Part model, mm, in its own coordinate system. Face numbers are marked on the shaded views. A direction names the side the tool comes from. Round coordinates to 2 decimals unless told otherwise and drop trailing zeros. Order: outer loops, then holes, each group sorted by start corner. A loop starts at its lowest first (then second) coordinate and runs counter-clockwise, first axis right, second up. Notation, with made-up numbers: (-33, 23) - (12, 23) arc R11 ccw to (12, 36) - close; hole circle Ø9 at (-14, -7). An arc over 180 degrees is marked (long way). Answer as a JSON object with one key per item and string values.
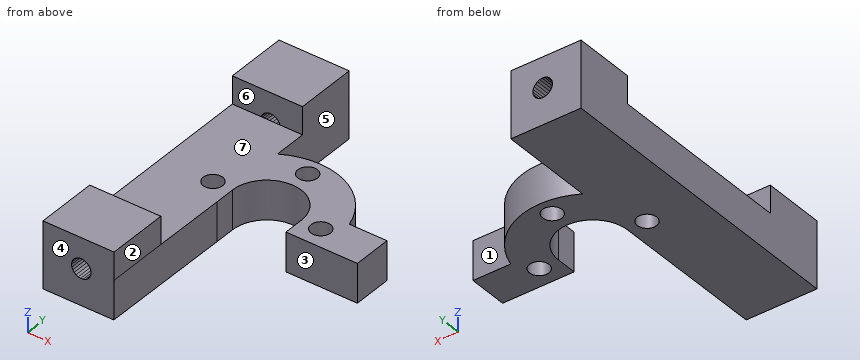
```python
from build123d import *

# Parameters (mm, degrees)
SKETCH1_R           = 1.5
BOSS_EXTRUDE1_DEPTH = 6
SKETCH2_W           = 10.807687298
SKETCH2_H           = 9.5
SKETCH2_W_2         = 10.943994224
BOSS_EXTRUDE2_DEPTH = 4.25
CUT_EXTRUDE1_DEPTH  = 9.5
CUT_EXTRUDE2_DEPTH  = 9.5


with BuildPart() as part:
    # Sketch1 → Boss-Extrude1 (new body)
    with BuildSketch(Plane.XY.offset(84.451608182)):
        with BuildLine():
            Line((40.02344809, 11.701998712), (40.02344809, 8.566491131))
            Line((40.02344809, 8.566491131), (47.02344809, 8.566491131))
            Line((47.02344809, 8.566491131), (51.02344809, 8.566491131))
            Line((51.02344809, 8.566491131), (51.02344809, 14.59568261))
            Line((51.02344809, 14.59568261), (45.222644144, 14.59568261))
            ThreePointArc((45.222644144, 14.59568261), (38.830062222, 21.788734788), (29.231135388, 21.10630759))
            Line((29.231135388, 21.10630759), (29.231135388, 35.703275576))
            Line((29.231135388, 35.703275576), (18.42344809, 35.703275576))
            Line((18.42344809, 35.703275576), (18.42344809, 14.59568261))
            Line((18.42344809, 14.59568261), (18.42344809, 8.566491131))
            Line((18.42344809, 8.566491131), (18.42344809, -12.296724841))
            Line((18.42344809, -12.296724841), (29.320619754, -12.296724841))
            Line((29.320619754, -12.296724841), (29.42344809, 8.566491131))
            Line((29.42344809, 8.566491131), (29.42344809, 11.701998712))
            ThreePointArc((29.42344809, 11.701998712), (34.72344809, 17.001998712), (40.02344809, 11.701998712))
        make_face()
        with Locations((43.02344809, 11.701998712)):
            Circle(SKETCH1_R, mode=Mode.SUBTRACT)
        with Locations((26.42344809, 11.701998712)):
            Circle(SKETCH1_R, mode=Mode.SUBTRACT)
        with Locations((34.72344809, 20.001998712)):
            Circle(SKETCH1_R, mode=Mode.SUBTRACT)
    extrude(amount=BOSS_EXTRUDE1_DEPTH)

    # Sketch2 → Boss-Extrude2 (add)
    with BuildSketch(Plane.XY.offset(90.451608182)):
        with Locations((23.827291739, 30.953275576)):
            Rectangle(SKETCH2_W, SKETCH2_H)
        with Locations((23.895445202, -7.546724841)):
            Rectangle(SKETCH2_W_2, SKETCH2_H)
    extrude(amount=BOSS_EXTRUDE2_DEPTH)

    # Sketch3 → Cut-Extrude1 (cut)
    with BuildSketch(Plane(origin=(0, 35.703275576, 0), x_dir=(1, 0, 0), z_dir=(0, 1, 0))):
        Polygon((24.039543919, -91.507423883), (24.414807311, -91.53103291), (24.784140042, -91.460577426), (25.124363355, -91.300484473), (25.414071731, -91.060813265), (25.635078303, -90.756623289), (25.773495189, -90.407027611), (25.820620111, -90.033992408), (25.773495189, -89.660958601), (25.635078303, -89.311362458), (25.414071731, -89.007172948), (25.124363355, -88.767500808), (24.784140042, -88.607407389), (24.414807311, -88.536952836), (24.039543919, -88.560561864), (23.681945852, -88.676751805), (23.364484064, -88.878222024), (23.107096306, -89.152314914), (22.925957791, -89.481805665), (22.832445554, -89.845992839), (22.832445554, -90.221992442), (22.925957791, -90.586179616), (23.107096306, -90.915670833), (23.364484064, -91.189762792), (23.681945852, -91.391233476), align=None)
    extrude(amount=-CUT_EXTRUDE1_DEPTH, mode=Mode.SUBTRACT)

    # Sketch4 → Cut-Extrude2 (cut)
    with BuildSketch(Plane.XZ.offset(12.296724841)):
        Polygon((25.27675753, 88.878222024), (24.959288291, 88.676751805), (24.601690225, 88.560561864), (24.226434282, 88.536952836), (23.857094101, 88.607407389), (23.516878239, 88.767500808), (23.227169863, 89.007172948), (23.00615584, 89.311362458), (22.867746405, 89.660958601), (22.820621482, 90.033992408), (22.867746405, 90.407027611), (23.00615584, 90.756623289), (23.227169863, 91.060813265), (23.516878239, 91.300484473), (23.857094101, 91.460577426), (24.226434282, 91.53103291), (24.601690225, 91.507423883), (24.959288291, 91.391233476), (25.27675753, 91.189762792), (25.534145287, 90.915670833), (25.715283803, 90.586179616), (25.80879604, 90.221992442), (25.80879604, 89.845992839), (25.715283803, 89.481805665), (25.534145287, 89.152314914), align=None)
    extrude(amount=-CUT_EXTRUDE2_DEPTH, mode=Mode.SUBTRACT)


solid = part.part
```
Item 1: Tool access for the marked faces 1, 2 and 3: list every direction of +Z, -Z, +X, -X, +Y, -Y with a clear straight run to the whole face (end or side of a thin tool).
Taken from the geometry:
{"face 1": "+Z, -Z, +X, +Y", "face 2": "+Z, -Z, +X, +Y, -Y", "face 3": "+Z, -Z, +X, -Y"}
Item 2: Cut at A-A (z = 92.75). Write the cut outline in (x, y), plus the area to 3 significant figures.
Taken from the geometry:
{"outline": "(18.42, -12.3) - (29.37, -12.3) - (29.37, -2.8) - (18.42, -2.8) - close; (18.42, 26.2) - (29.23, 26.2) - (29.23, 35.7) - (18.42, 35.7) - close", "area": "207 mm2"}
Item 3: Drop flat-ended pins along their axis: P1, Ø3.5, axis at y = -6, z = 92.5, coming from the +X side; P2, Ø2, axis at x = 34.5, z = 88, coming from the -Y side; P3, Ø8, axis at x = 25, y = 25.5, coming from the +Z side; P4, Ø4.5, axis at x = 49, z = 88.5, coming from the +Y side. Give the stop position or say it passes through.
Taken from the geometry:
{"P1": "x = 29.37", "P2": "y = 16.86", "P3": "z = 94.7", "P4": "y = 14.6"}
Item 4: Two-plate mould, pull along Y, no slides. Class the marked faces 4, 5, 6 and 7: pulls with the +Y half, pulls with the -Y half, needs draft (parallel to the pull), parting line crosses it, or undercut.
Taken from the geometry:
{"face 4": "pulls with the -Y half", "face 5": "needs draft", "face 6": "undercut", "face 7": "undercut"}
Item 5: Probe L1, parallel to Y at x = 26, z = 92; L2, parallel to X at y = 28, z = 89.5; L3, parallel to X at y = 10, z = 88.75. List the from-to ranges inside material, lowest first. Write a range as from..to.
Taken from the geometry:
{"L1": "-12.3..-2.8, 26.2..35.7", "L2": "18.42..22.92, 25.71..29.23", "L3": "18.42..29.42, 40.02..51.02"}
Item 6: Cut at D-D (y = 16.5). Write the cut outline in (x, z).
Taken from the geometry:
{"outline": "(18.42, 84.45) - (32.47, 84.45) - (32.47, 90.45) - (18.42, 90.45) - close; (36.97, 84.45) - (44.5, 84.45) - (44.5, 90.45) - (36.97, 90.45) - close"}
Item 7: Cut at C-C (x = 27). Write the cut outline in (y, z).
Taken from the geometry:
{"outline": "(-12.3, 84.45) - (10.32, 84.45) - (10.32, 90.45) - (-2.8, 90.45) - (-2.8, 94.7) - (-12.3, 94.7) - close; (13.09, 84.45) - (35.7, 84.45) - (35.7, 94.7) - (26.2, 94.7) - (26.2, 90.45) - (13.09, 90.45) - close"}
